Part print with two shaded views. Sizes in mm from the minimum x, y, z corner. A direction names the side the tool comes from. Round coordinates to 2 decimals unless told otherwise and drop trailing zeros. Loops run counter-clockwise (first coordinate to the right, second up) from the corner with the lowest first, then second, coordinate; pieces in that order, holes last. Notation, with made-up numbers: (-21, 79) -> (26, 79) arc R35 cw to (26, 117) -> close; hole circle Ø10 at (30, -38.5). An arc over 180 degrees is marked (long way). Use a Markdown table: item, result. Add a question column.
Item 1: Probe line 1 (Y direction, x = 136, z = 71); line 2 (X direction, y = 15, z = 41.5); line 3 (X direction, y = 80, z = 43). List the from-to ranges inside material, lowest first. Write a range as [from, to].
Item 2: Flat gauge pins, fed straight in: pin 1 (2 mm diameter, centred on y = 76, z = 32, fed in from -X); pin 2 (2.5 mm diameter, centred on y = 135.5, z = 108, fed in from -X); pin 3 (0.9 mm diameter, centred on x = 61.5, y = 135.5, fed in from +Z). Where does each tip first touch, or does it go through?
Item 3: Cut at A-A, the plane z = 122. List the corners of the cut face in (x, y).
Item 4: Which spindle directions (+Z, -Z, +X, -X, +Y, -Y) get a long thin tool onto all of the face, cutting with end or side? Do the marked faces 1 and 2. Say none if no direction does.
Item 5: Cut at D-D, the plane z = 89. List the corners of the cut face in (x, y).
Item 6: Cut at B-B, the plane y = 119. List the corners of the cut face in (x, z).
Item 7: Cut at C-C, the plane x = 118. List the corners of the cut face in (y, z), plus the area to 3 significant figures.
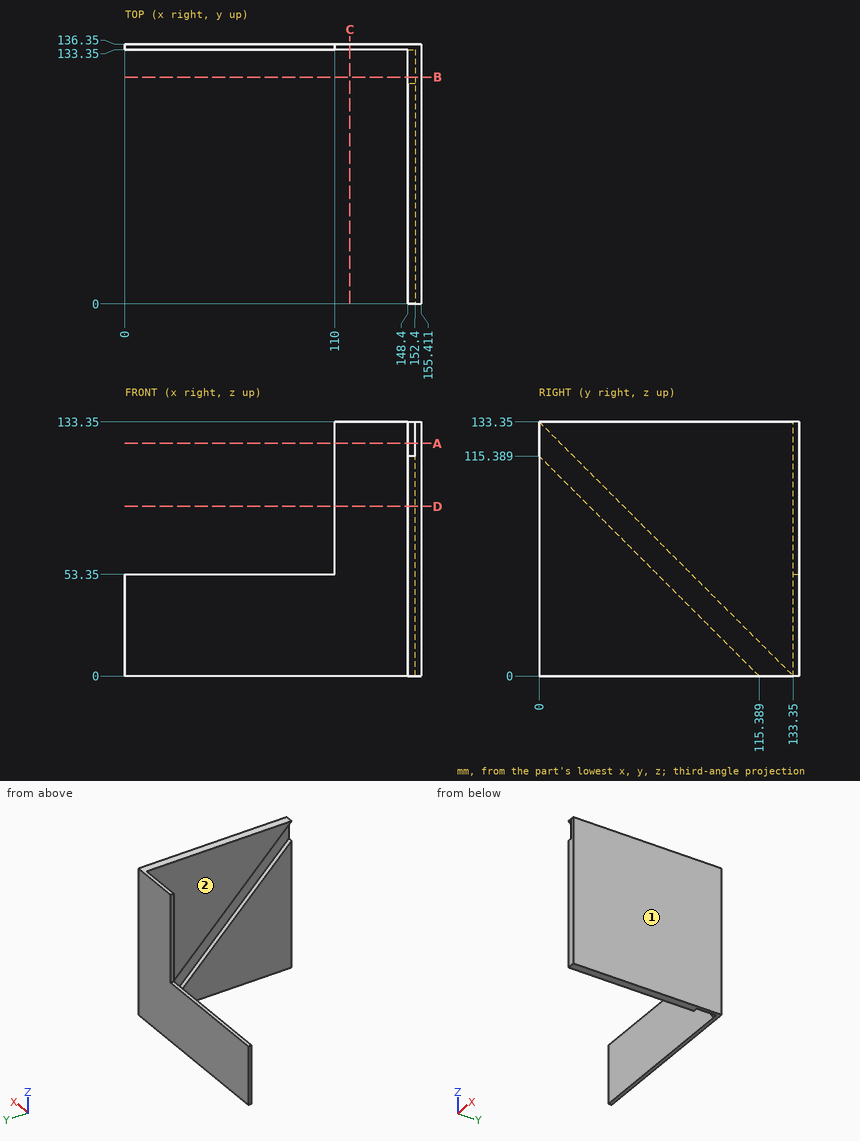
A:
| question | item | result |
|---|---|---|
| 1 | line 1 | y = [133.35, 136.35] |
| 1 | line 2 | x = [148.4, 155.41] |
| 1 | line 3 | x = [152.4, 155.41] |
| 2 | pin 1 | stops at x = 148.4 |
| 2 | pin 2 | stops at x = 110 |
| 2 | pin 3 | stops at z = 53.35 |
| 3 | outline | (110, 133.35) -> (148.4, 133.35) -> (148.4, 11.35) -> (152.4, 11.35) -> (152.4, 0) -> (155.41, 0) -> (155.41, 136.35) -> (110, 136.35) -> close |
| 4 | face 1 | +Z, -Z, +X, +Y, -Y |
| 4 | face 2 | +Z, -Z, -X, -Y |
| 5 | outline | (110, 133.35) -> (148.4, 133.35) -> (148.4, 44.35) -> (152.4, 44.35) -> (152.4, 26.39) -> (148.4, 26.39) -> (148.4, 0) -> (155.41, 0) -> (155.41, 136.35) -> (110, 136.35) -> close |
| 6 | outline | (148.4, 14.35) -> (152.4, 14.35) -> (152.4, 0) -> (155.41, 0) -> (155.41, 133.35) -> (148.4, 133.35) -> close |
| 7 | outline | (133.35, 0) -> (136.35, 0) -> (136.35, 133.35) -> (133.35, 133.35) -> close |
| 7 | area | 400 mm^2 |
